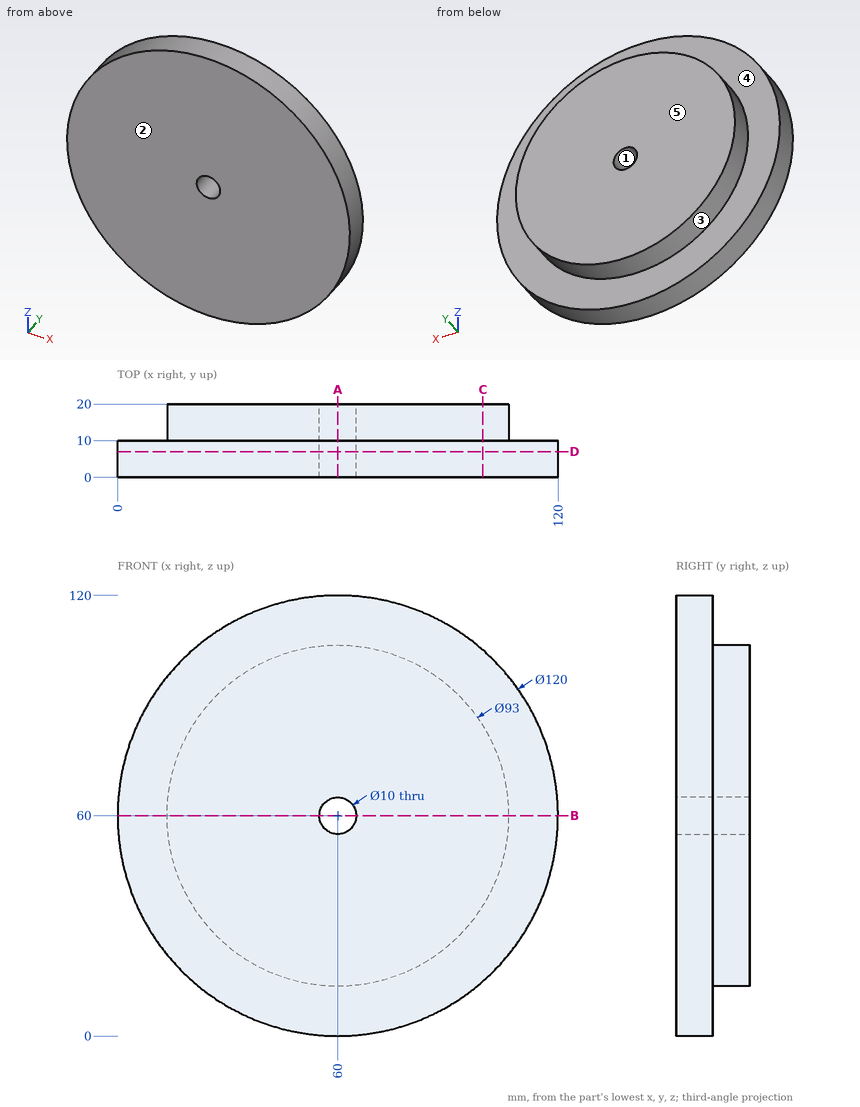
Job drawing, mm, ordinate dimensions from the low corner. One solid piece. A direction names the side the tool comes from. Round coordinates to 2 decimals unless told otherwise and drop trailing zeros. Write each loop counter-clockwise with the first axis right and the second up, starting at its lowest first coordinate (ties: lowest second). Pieces come first, ordered by that corner, then holes. Notation, with made-up numbers: M -33,58 L -18,58 A32 cw -18,93 Z; hole C 89.5,-3 d9. An arc over 180 degrees is marked long. Return JSON: item names as keys, results as strings. Group by question number.
(1) Pin check, flat tips, straight feed: pin 1 Ø5 at (x, y) = (49.5, 14.5) entering from -Z; pin 2 Ø12 at (x, y) = (49, 8.5) entering from -Z; pin 3 Ø3 at (x, y) = (65, 6.5) entering from -Z. Stop position of each tip, or through.
(2) Saw through at A-A on x = 60. Write the cut outline in (y, z).
(3) Drill centre lines: probe 1 along X at (y, z) = (13, 60); probe 2 along X at (y, z) = (8, 60); probe 3 along Z at (x, y) = (63, 9.5). Where is each one in solid material? Low to high.
(4) Saw through at D-D on y = 7. Write the cut outline in (x, z).
(5) Which spindle directions (+Z, -Z, +X, -X, +Y, -Y) get a long thin tool onto all of the face, cutting with end or side? Do the marked faces 4 and 5. Say none if no direction does.
(6) Two-plate mould, pull along Z, no slides. Class the marked faces 1, 2 and 3: +Z half, -Z half, draft (parallel to the pull), parting line (faces both ways), or undercut.
(7) Saw through at C-C on x = 99.5. Write the cut outline in (y, z).
(8) Saw through at B-B on z = 60. Write the cut outline in (x, y).
Returned:
{
 "1": {"pin 1": "z = 14.19", "pin 2": "z = 0.21", "pin 3": "z = 0.1"},
 "2": {"outline": "M 0,0 L 10,0 L 10,13.5 L 20,13.5 L 20,55 L 0,55 Z; M 0,65 L 20,65 L 20,106.5 L 10,106.5 L 10,120 L 0,120 Z"},
 "3": {"probe 1": "13.5 to 55, 65 to 106.5", "probe 2": "0 to 55, 65 to 120", "probe 3": "0.08 to 56, 64 to 119.92"},
 "4": {"outline": "C 60,60 d120; hole C 60,60 d10"},
 "5": {"face 4": "+Y", "face 5": "+Z, -Z, +X, -X, +Y"},
 "6": {"face 1": "undercut", "face 2": "draft", "face 3": "parting line"},
 "7": {"outline": "M 0,14.84 L 10,14.84 L 10,35.46 L 20,35.46 L 20,84.54 L 10,84.54 L 10,105.16 L 0,105.16 Z"},
 "8": {"outline": "M 0,0 L 55,0 L 55,20 L 13.5,20 L 13.5,10 L 0,10 Z; M 65,0 L 120,0 L 120,10 L 106.5,10 L 106.5,20 L 65,20 Z"}
}
